Source: CAD feature listing. Evaluate the final solid. Frame: model axes, mm. Face numbers are marked on the shaded views. Coordinates: 2 decimals unless noted, no trailing zeros. Loops run counter-clockwise (first coordinate to the right, second up) from the corner with the lowest first, then second, coordinate; pieces in that order, holes last.
Item 1: Line query: probe 1 along Z at (x, y) = (8, -20.5); probe 2 along Z at (x, y) = (8, -10.5); probe 3 along Y at (x, z) = (-5, 5.25). Output: solid intervals per line, ascending.
Item 2: Section query B-B, the plane x = 12.5. Return the cut outline in (y, z).
Item 3: Pin query (flat end, axial travel): pin 1 Ø1 at (x, z) = (-5.5, 7) entering from -Y; pin 2 Ø5 at (y, z) = (-19.5, 6.5) entering from -X; pin 3 Ø2 at (x, z) = (2.5, 9.5) entering from +Y; pin 4 Ø1.2 at (x, y) = (-3.5, -19.5) entering from -Z. Return the tip coordinate at first contact, or that it passes through.
Item 4: Pull-direction query (Z, two-part tool) for the marked faces 1, 2 and 3; classes: +Z half, -Z half, draft (parallel to the pull), parting line (faces both ways), or undercut.
Item 5: Section query C-C, the plane x = 2.5. Return the cut outline in (y, z).
Item 6: Section query D-D, the plane y = -23. Return the cut outline in (x, z), then the cut area to 3 significant figures.
Item 7: Section query A-A, the plane y = 0. Return the cut outline in (x, z), then the cut area to 3 significant figures.
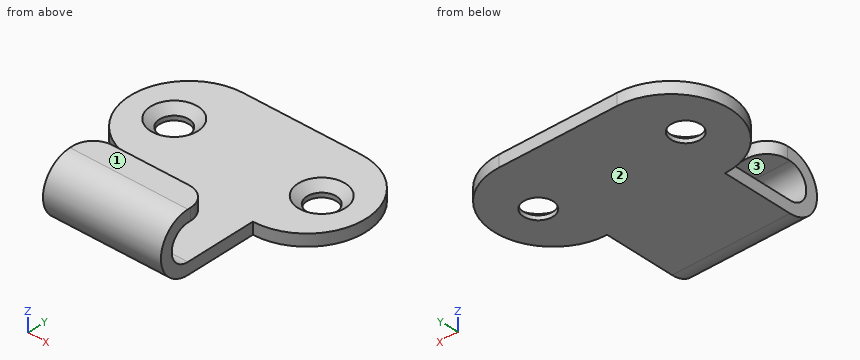
```python
from build123d import *

# Parameters (mm, degrees)
T_LE_DE_BASE_PLI_E1_DEPTH = 10
PATTE1_DEPTH              = 2
ESQUISSE9_R               = 2.5
ENL_V_MAT_EXTRU_1_DEPTH   = 35.539832078
CHANFREIN1_SIZE           = 1.5
CHANFREIN1_SIZE2          = 1.258649447
CONG_1_R                  = 3.5


# Sheet-metal steps are written as plain solids
with BuildPart() as part:
    # Esquisse1 → Tôle de base pliée1 (new, symmetric)
    with BuildSketch(Plane(origin=(0, 0, 0), x_dir=(0, 0, -1), z_dir=(1, 0, 0))):
        with BuildLine():
            Line((0, 10), (0, -22))
            ThreePointArc((0, -22), (-5, -27), (-10, -22))
            Line((-10, -22), (-10, -18))
            Line((-10, -18), (-8, -18))
            Line((-8, -18), (-8, -22))
            ThreePointArc((-8, -22), (-5, -25), (-2, -22))
            Line((-2, -22), (-2, 10))
            Line((-2, 10), (0, 10))
        make_face()
    extrude(amount=T_LE_DE_BASE_PLI_E1_DEPTH, both=True)

    # Esquisse6 → Patte1 (add)
    with BuildSketch(Plane.XY.offset(2)):
        with BuildLine():
            Line((-10, 10), (10, 10))
            ThreePointArc((10, 10), (20, 0), (10, -10))
            Line((10, -10), (-10, -10))
            ThreePointArc((-10, -10), (-20, 0), (-10, 10))
        make_face()
    extrude(amount=-PATTE1_DEPTH)

    # Esquisse9 → Enlèv. mat.-Extru.1 (cut, through all)
    with BuildSketch(Plane.XY.offset(2)):
        with Locations((-12.5, 0)):
            Circle(ESQUISSE9_R)
        with Locations(Location((12.5, 0, 0), (0, 0, 180))):
            Circle(ESQUISSE9_R)
    extrude(amount=-ENL_V_MAT_EXTRU_1_DEPTH, mode=Mode.SUBTRACT)

    # Chanfrein1
    chanfrein1_edges = [part.edges().sort_by_distance(p)[0] for p in [
        (-15, 0, 2),
        (15, 0, 2),
    ]]
    chanfrein1_side = [part.faces().sort_by_distance(p)[0] for p in [
        (0, -4.197228845, 2),
    ]]
    chamfer(chanfrein1_edges, length=CHANFREIN1_SIZE, length2=CHANFREIN1_SIZE2, reference=chanfrein1_side[0])

    # Congé1
    cong_1_edges = [part.edges().sort_by_distance(p)[0] for p in [
        (10, -18, 9),
        (-10, -18, 9),
    ]]
    fillet(cong_1_edges, radius=CONG_1_R)


solid = part.part
```
Verdict:
1. probe 1: z = 0 to 2, 8 to 10
1. probe 2: z = 0 to 2
1. probe 3: y = -26.99 to -24.99
2. outline: (-9.68, 0) - (-2.5, 0) - (-2.5, 0.74) - (-4, 2) - (-9.68, 2) - close; (2.5, 0) - (9.68, 0) - (9.68, 2) - (4, 2) - (2.5, 0.74) - close
3. pin 1: stops at y = -26.77
3. pin 2: stops at x = -10
3. pin 3: stops at y = -18
3. pin 4: stops at z = 0
4. face 1: +Z half
4. face 2: -Z half
4. face 3: undercut
5. outline: (-22, 0) - (10, 0) - (10, 2) - (-22, 2) arc R3 cw to (-22, 8) - (-18, 8) - (-18, 10) - (-22, 10) arc R5 ccw to start
6. outline: (-10, 0.1) - (10, 0.1) - (10, 2.17) - (-10, 2.17) - close; (-10, 7.83) - (10, 7.83) - (10, 9.9) - (-10, 9.9) - close
6. area: 82.8 mm2
7. outline: (-20, 0) - (-15, 0) - (-15, 0.74) - (-16.5, 2) - (-20, 2) - close; (-10, 0) - (10, 0) - (10, 0.74) - (8.5, 2) - (-8.5, 2) - (-10, 0.74) - close; (15, 0) - (20, 0) - (20, 2) - (16.5, 2) - (15, 0.74) - close
7. area: 56.2 mm2
